Geometry check sheet. Reference: the model listing, model coordinates, mm. Face numbers are marked on the shaded views. A direction names the side the tool comes from. Give positions to 0.01 mm unless a question says otherwise; leave off trailing zeros. Write each loop counter-clockwise with the first axis right and the second up, starting at its lowest first coordinate (ties: lowest second). Pieces come first, ordered by that corner, then holes. Notation, with made-up numbers: M -12.5,-32 L 17.5,-32 A3 cw 17.5,-27 Z; hole C -4,-36.5 d1. An arc over 180 degrees is marked long. One line per item, written item: value. Start each with the question number.
1. Release check for a two-part mould opening along X. For the marked faces 1, 2, 3 and 4 record: pulls with the +X half, pulls with the -X half, needs draft (parallel to the pull), parting line crosses it, or undercut.
2. Gauge pin test, flat ends, axial feed: pin 1 (1.6 mm diameter, centred on x = -7.5, y = -4.5, fed in from -Z); pin 2 (1 mm diameter, centred on x = 8.5, z = 42.5, fed in from -Y); pin 3 (10 mm diameter, centred on y = 1, z = 49.5, fed in from -X); pin 4 (1.5 mm diameter, centred on x = -5, y = -12.5, fed in from -Z). Record the tip position at first contact, or that the pin passes through.
3. Cross-section at B-B on x = 0. Record the cut outline in (y, z), then the cut area to 4 significant figures.
4. Scan lines: line 1 (Y direction, x = 0, z = 47.95); line 2 (Y direction, x = 0, z = 17.5); line 3 (Z direction, x = 5, y = 15). Record each from-to range of solid material in increasing order.
5. Cross-section at A-A on y = 0. Record the cut outline in (x, z), then the cut area to 4 significant figures.
6. Cross-section at D-D on x = 4. Record the cut outline in (y, z).
7. Tool access check on the marked faces 5, 6, 7 and 8. Record the directions out of +Z, -Z, +X, -X, +Y, -Y that give a thin tool (end or side, any length) a straight path to the whole face; none if there is none.
8. Cross-section at C-C on z = 20. Record the cut outline in (x, y).
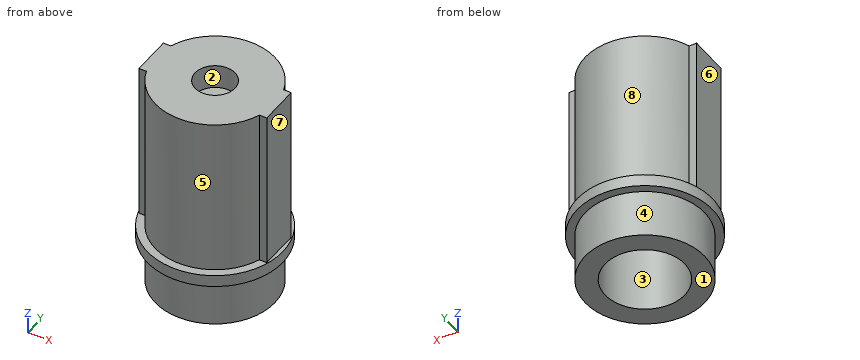
from build123d import *

# Parameters (mm, degrees)
SKETCH1_R           = 15
BOSS_EXTRUDE1_DEPTH = 55
SKETCH2_R           = 10
CUT_EXTRUDE7_DEPTH  = 46
SKETCH7_R           = 5
CUT_EXTRUDE8_DEPTH  = 6
SKETCH8_R           = 2.25
CUT_EXTRUDE9_DEPTH  = 3
BOSS_EXTRUDE5_START = 6
BOSS_EXTRUDE5_DEPTH = 6
BOSS_EXTRUDE6_START = -3
SKETCH11_R          = 17
SKETCH11_R_2        = 15
BOSS_EXTRUDE6_DEPTH = 3
BOSS_EXTRUDE8_START = -40
BOSS_EXTRUDE8_DEPTH = 40


with BuildPart() as part:
    # Sketch1 → Boss-Extrude1 (new body)
    with BuildSketch(Plane.XY):
        Circle(SKETCH1_R)
    extrude(amount=BOSS_EXTRUDE1_DEPTH)

    # Sketch2 → Cut-Extrude7 (cut)
    with BuildSketch(Plane(origin=(0, 0, 0), x_dir=(-1, 0, 0), z_dir=(0, 0, -1))):
        Circle(SKETCH2_R)
    extrude(amount=-CUT_EXTRUDE7_DEPTH, mode=Mode.SUBTRACT)

    # Sketch7 → Cut-Extrude8 (cut)
    with BuildSketch(Plane.XY.offset(55)):
        Circle(SKETCH7_R)
    extrude(amount=-CUT_EXTRUDE8_DEPTH, mode=Mode.SUBTRACT)

    # Sketch8 → Cut-Extrude9 (cut)
    with BuildSketch(Plane.XY.offset(49)):
        Circle(SKETCH8_R)
    extrude(amount=-CUT_EXTRUDE9_DEPTH, mode=Mode.SUBTRACT)

    # Sketch9 → Boss-Extrude5 (add)
    with BuildSketch(Plane(origin=(0, 0, 46), x_dir=(-1, 0, 0), z_dir=(0, 0, -1)).offset(BOSS_EXTRUDE5_START)):
        with BuildLine():
            Line((-9.682458366, -2.5), (-6.5, -2.5))
            Line((-6.5, -2.5), (-6.5, -7.599342077))
            ThreePointArc((-6.5, -7.599342077), (-8.48344341, -5.294448782), (-9.682458366, -2.5))
        make_face()
        with BuildLine():
            Line((-9.682458366, 2.5), (-6.5, 2.5))
            Line((-6.5, 2.5), (-6.5, 7.599342077))
            ThreePointArc((-6.5, 7.599342077), (-8.48344341, 5.294448782), (-9.682458366, 2.5))
        make_face()
        with BuildLine():
            Line((9.682458366, -2.5), (6.5, -2.5))
            Line((6.5, -2.5), (6.5, -7.599342077))
            ThreePointArc((6.5, -7.599342077), (8.48344341, -5.294448782), (9.682458366, -2.5))
        make_face()
        with BuildLine():
            Line((6.5, 2.5), (6.5, 7.599342077))
            ThreePointArc((6.5, 7.599342077), (8.48344341, 5.294448782), (9.682458366, 2.5))
            Line((9.682458366, 2.5), (6.5, 2.5))
        make_face()
    extrude(amount=-BOSS_EXTRUDE5_DEPTH)

    # Sketch11 → Boss-Extrude6 (add)
    with BuildSketch(Plane.XY.offset(15).offset(BOSS_EXTRUDE6_START)):
        Circle(SKETCH11_R)
        Circle(SKETCH11_R_2, mode=Mode.SUBTRACT)
    extrude(amount=BOSS_EXTRUDE6_DEPTH)

    # Sketch10 → Boss-Extrude8 (add)
    with BuildSketch(Plane.XY.offset(55).offset(BOSS_EXTRUDE8_START)):
        with BuildLine():
            Line((16, 5), (14.142135624, 5))
            ThreePointArc((14.142135624, 5), (15, 0), (14.142135624, -5))
            Line((14.142135624, -5), (16, -5))
            Line((16, -5), (16, 5))
        make_face()
        with BuildLine():
            ThreePointArc((-14.142135624, 5), (-15, 0), (-14.142135624, -5))
            Line((-14.142135624, -5), (-16, -5))
            Line((-16, -5), (-16, 5))
            Line((-16, 5), (-14.142135624, 5))
        make_face()
    extrude(amount=BOSS_EXTRUDE8_DEPTH)


solid = part.part
Report:
1. face 1: needs draft
1. face 2: undercut
1. face 3: undercut
1. face 4: parting line crosses it
2. pin 1: stops at z = 40
2. pin 2: stops at y = -12.69
2. pin 3: stops at x = -16
2. pin 4: stops at z = 0
3. outline: M -17,12 L -15,12 L -15,0 L -10,0 L -10,46 L -2.25,46 L -2.25,49 L -5,49 L -5,55 L -15,55 L -15,15 L -17,15 Z; M 2.25,46 L 10,46 L 10,0 L 15,0 L 15,12 L 17,12 L 17,15 L 15,15 L 15,55 L 5,55 L 5,49 L 2.25,49 Z
3. area: 668.5 mm^2
4. line 1: y = -15 to -2.25, 2.25 to 15
4. line 2: y = -15 to -10, 10 to 15
4. line 3: z = 12 to 15
5. outline: M -17,12 L -15,12 L -15,0 L -10,0 L -10,46 L -2.25,46 L -2.25,49 L -5,49 L -5,55 L -16,55 L -16,15 L -17,15 Z; M 2.25,46 L 10,46 L 10,0 L 15,0 L 15,12 L 17,12 L 17,15 L 16,15 L 16,55 L 5,55 L 5,49 L 2.25,49 Z
5. area: 748.5 mm^2
6. outline: M -16.52,12 L -14.46,12 L -14.46,0 L -9.17,0 L -9.17,46 L 9.17,46 L 9.17,0 L 14.46,0 L 14.46,12 L 16.52,12 L 16.52,15 L 14.46,15 L 14.46,55 L 3,55 L 3,49 L -3,49 L -3,55 L -14.46,55 L -14.46,15 L -16.52,15 Z
7. face 5: +Z, -Y
7. face 6: +Z, -X, +Y, -Y
7. face 7: +Z, +X, +Y, -Y
7. face 8: +Z, +Y
8. outline: M -16,-5 L -14.14,-5 A15 ccw 14.14,-5 L 16,-5 L 16,5 L 14.14,5 A15 ccw -14.14,5 L -16,5 Z; hole C 0,0 d20
